The listing builds one solid part. Answer for the finished solid, in the listing's coordinates (mm). Give positions to 0.01 mm unless a question says otherwise; leave off trailing zeros. Loops run counter-clockwise (first coordinate to the right, second up) from the corner with the lowest first, then second, coordinate; pieces in that order, holes last.
Item 1: Section A-A, the plane z = 0 is taken. Give the vertices of the cut face in (x, y) (3 decimals), and give its area (3 significant figures).
Item 2: Consider line 1 along X through (y, z) = (58, 0) (3 decimals); line 2 along Z through (x, y) = (6, 59); line 3 along Y through (x, z) = (-28, 7). Determine where each line is inside the solid, lowest interval first.
Item 3: Each of these flat-tipped pins is pushed along its axis until it touches: pin 1 Ø3 at (x, z) = (7, -1.5) entering from +Y; pin 2 Ø1.6 at (x, y) = (19.68, -67.47) entering from +Z; pin 3 Ø10 at (x, z) = (-6.35, 0) entering from +Y. Where does it stop, or does it pass through?
Item 4: Section B-B, the plane x = -6.35 is taken. Give the vertices of the cut face in (y, z) (3 decimals).
from build123d import *

# Parameters (mm, degrees)
SKETCH1_W           = 82.55
SKETCH1_H           = 173.0375
BOSS_EXTRUDE1_DEPTH = 19.05
SKETCH2_R           = 0.889
CUT_EXTRUDE1_DEPTH  = 104.153912803
FILLET1_R           = 2.54
SKETCH3_R           = 3.175
CUT_EXTRUDE2_DEPTH  = 50.8


with BuildPart() as part:
    # Sketch1 → Boss-Extrude1 (new, symmetric)
    with BuildSketch(Plane.XY):
        Rectangle(SKETCH1_W, SKETCH1_H)
    extrude(amount=BOSS_EXTRUDE1_DEPTH, both=True)

    # Sketch2 → Cut-Extrude1 (cut, through all)
    with BuildSketch(Plane.XY.offset(19.05)):
        with Locations((-28.575, -67.46875)):
            Circle(SKETCH2_R)
        with Locations((-19.685, -67.46875)):
            Circle(SKETCH2_R)
        with Locations((28.575, -67.46875)):
            Circle(SKETCH2_R)
        with Locations((19.685, -67.46875)):
            Circle(SKETCH2_R)
    extrude(amount=-CUT_EXTRUDE1_DEPTH, mode=Mode.SUBTRACT)

    # Fillet1
    fillet1_edges = [part.edges().sort_by_distance(p)[0] for p in [
        (-41.275, 0, 19.05),
        (41.275, 0, 19.05),
        (-41.275, 0, -19.05),
        (41.275, 0, -19.05),
    ]]
    fillet(fillet1_edges, radius=FILLET1_R)

    # Sketch3 → Cut-Extrude2 (cut)
    with BuildSketch(Plane(origin=(0, 86.51875, 0), x_dir=(1, 0, 0), z_dir=(0, 1, 0))):
        with Locations(Location((19.05, 0, 0), (0, 0, 270))):
            Circle(SKETCH3_R)
        with Locations(Location((-19.05, 0, 0), (0, 0, 270))):
            Circle(SKETCH3_R)
        with Locations(Location((-6.35, 0, 0), (0, 0, 270))):
            Circle(SKETCH3_R)
        with Locations(Location((6.35, 0, 0), (0, 0, 270))):
            Circle(SKETCH3_R)
    extrude(amount=-CUT_EXTRUDE2_DEPTH, mode=Mode.SUBTRACT)


solid = part.part
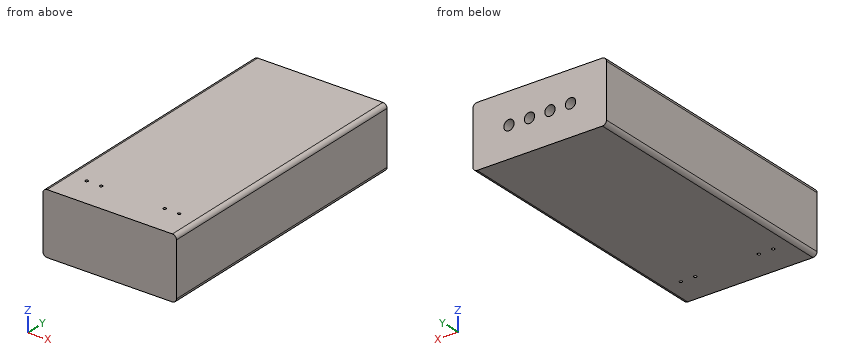
Worked answers:
1. outline: (-41.275, -86.519) - (41.275, -86.519) - (41.275, 86.519) - (22.225, 86.519) - (22.225, 35.719) - (15.875, 35.719) - (15.875, 86.519) - (9.525, 86.519) - (9.525, 35.719) - (3.175, 35.719) - (3.175, 86.519) - (-3.175, 86.519) - (-3.175, 35.719) - (-9.525, 35.719) - (-9.525, 86.519) - (-15.875, 86.519) - (-15.875, 35.719) - (-22.225, 35.719) - (-22.225, 86.519) - (-41.275, 86.519) - close; hole circle Ø1.778 at (-28.575, -67.469); hole circle Ø1.778 at (-19.685, -67.469); hole circle Ø1.778 at (19.685, -67.469); hole circle Ø1.778 at (28.575, -67.469)
1. area: 13,000 mm2
2. line 1: x = -41.275 to -22.225, -15.875 to -9.525, -3.175 to 3.175, 9.525 to 15.875, 22.225 to 41.275
2. line 2: z = -19.05 to -3.16, 3.16 to 19.05
2. line 3: y = -86.52 to -68.15, -66.79 to 86.52
3. pin 1: stops at y = 35.72
3. pin 2: passes through
3. pin 3: stops at y = 86.52
4. outline: (-86.519, -19.05) - (86.519, -19.05) - (86.519, -3.175) - (35.719, -3.175) - (35.719, 3.175) - (86.519, 3.175) - (86.519, 19.05) - (-86.519, 19.05) - close
